from build123d import *

# Parameters (mm, degrees)
F0_R     = 12.7
F1_DEPTH = 6.35
F0_W     = 1.27
F0_H     = 1.27
F2_DEPTH = 2.794


with BuildPart() as f1:
    # F0 (on Front) → F1 (new body, symmetric)
    with BuildSketch(Plane.XZ):
        Circle(F0_R)
        with BuildLine():
            ThreePointArc((8.1567226875, 1.27), (8.2303939998, 0.636898428), (8.255, 0))
            ThreePointArc((8.255, 0), (8.2303939998, -0.636898428), (8.1567226875, -1.27))
            ThreePointArc((8.1567226875, -1.27), (5.8371664787, -5.8371664787), (1.27, -8.1567226875))
            ThreePointArc((1.27, -8.1567226875), (0.636898428, -8.2303939998), (0, -8.255))
            ThreePointArc((0, -8.255), (-0.636898428, -8.2303939998), (-1.27, -8.1567226875))
            ThreePointArc((-1.27, -8.1567226875), (-5.8371664787, -5.8371664787), (-8.1567226875, -1.27))
            ThreePointArc((-8.1567226875, -1.27), (-8.2303939998, -0.636898428), (-8.255, 0))
            ThreePointArc((-8.255, 0), (-8.2303939998, 0.636898428), (-8.1567226875, 1.27))
            ThreePointArc((-8.1567226875, 1.27), (-5.8371664787, 5.8371664787), (-1.27, 8.1567226875))
            ThreePointArc((-1.27, 8.1567226875), (-0.636898428, 8.2303939998), (0, 8.255))
            ThreePointArc((0, 8.255), (0.636898428, 8.2303939998), (1.27, 8.1567226875))
            ThreePointArc((1.27, 8.1567226875), (5.8371664787, 5.8371664787), (8.1567226875, 1.27))
        make_face(mode=Mode.SUBTRACT)
    extrude(amount=F1_DEPTH, both=True)

    # F0 (on Front) → F2 (join, symmetric)
    with BuildSketch(Plane.XZ):
        with BuildLine():
            Line((1.27, 1.27), (1.27, 8.1567226875))
            ThreePointArc((1.27, 8.1567226875), (0.636898428, 8.2303939998), (0, 8.255))
            Line((0, 8.255), (0, 1.27))
            Line((0, 1.27), (1.27, 1.27))
        make_face()
        with BuildLine():
            Line((0, 1.27), (0, 8.255))
            ThreePointArc((0, 8.255), (-0.636898428, 8.2303939998), (-1.27, 8.1567226875))
            Line((-1.27, 8.1567226875), (-1.27, 1.27))
            Line((-1.27, 1.27), (0, 1.27))
        make_face()
        with Locations((-0.635, 0.635)):
            Rectangle(F0_W, F0_H)
        with Locations((0.635, 0.635)):
            Rectangle(F0_W, F0_H)
        with Locations((0.635, -0.635)):
            Rectangle(F0_W, F0_H)
        with Locations((-0.635, -0.635)):
            Rectangle(F0_W, F0_H)
        with BuildLine():
            ThreePointArc((-1.27, -8.1567226875), (-0.636898428, -8.2303939998), (0, -8.255))
            Line((0, -8.255), (0, -1.27))
            Line((0, -1.27), (-1.27, -1.27))
            Line((-1.27, -1.27), (-1.27, -8.1567226875))
        make_face()
        with BuildLine():
            ThreePointArc((0, -8.255), (0.636898428, -8.2303939998), (1.27, -8.1567226875))
            Line((1.27, -8.1567226875), (1.27, -1.27))
            Line((1.27, -1.27), (0, -1.27))
            Line((0, -1.27), (0, -8.255))
        make_face()
        with BuildLine():
            Line((-8.255, 0), (-1.27, 0))
            Line((-1.27, 0), (-1.27, 1.27))
            Line((-1.27, 1.27), (-8.1567226875, 1.27))
            ThreePointArc((-8.1567226875, 1.27), (-8.2303939998, 0.636898428), (-8.255, 0))
        make_face()
        with BuildLine():
            Line((-1.27, -1.27), (-1.27, 0))
            Line((-1.27, 0), (-8.255, 0))
            ThreePointArc((-8.255, 0), (-8.2303939998, -0.636898428), (-8.1567226875, -1.27))
            Line((-8.1567226875, -1.27), (-1.27, -1.27))
        make_face()
        with BuildLine():
            ThreePointArc((8.1567226875, -1.27), (8.2303939998, -0.636898428), (8.255, 0))
            Line((8.255, 0), (1.27, 0))
            Line((1.27, 0), (1.27, -1.27))
            Line((1.27, -1.27), (8.1567226875, -1.27))
        make_face()
        with BuildLine():
            Line((1.27, 0), (8.255, 0))
            ThreePointArc((8.255, 0), (8.2303939998, 0.636898428), (8.1567226875, 1.27))
            Line((8.1567226875, 1.27), (1.27, 1.27))
            Line((1.27, 1.27), (1.27, 0))
        make_face()
    extrude(amount=F2_DEPTH, both=True)


solid = f1.part
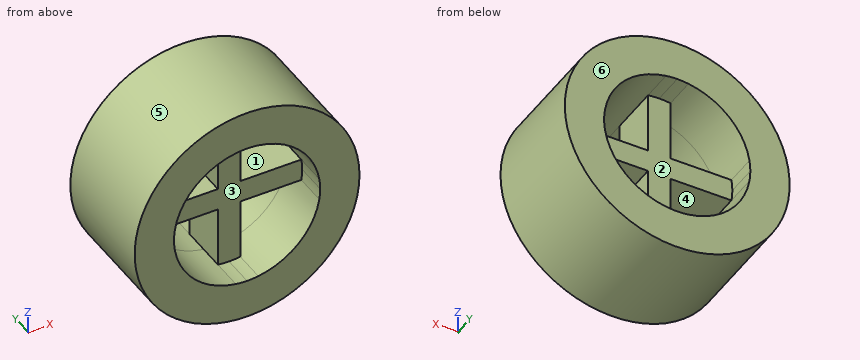
For this review, take the finished solid that the model builds, in its own axes (mm). Face numbers are marked on the shaded views. A direction names the side the tool comes from. Round coordinates to 2 decimals unless told otherwise and drop trailing zeros. Loops run counter-clockwise (first coordinate to the right, second up) from the corner with the lowest first, then second, coordinate; pieces in that order, holes last. Notation, with made-up numbers: (31.5, -32) - (83.5, -32) arc R36 cw to (83.5, 7) - close; hole circle Ø8 at (74.5, 8). An arc over 180 degrees is marked (long way). Use one line per item in the form item = value.
Item 1: Mouldability with a two-part tool opening along Z and no side actions: class the marked faces 4, 5 and 6 as +Z half, -Z half, draft (parallel to the pull), parting line (faces both ways), or undercut.
Answers:
face_4 = undercut
face_5 = parting line
face_6 = draft
Item 2: Consider section B-B on x = 2.5. Write out the cut boundary in (y, z), then the cut area to 3 significant figures.
Answers:
outline = (-6.35, -12.45) - (6.35, -12.45) - (6.35, -7.87) - (-6.35, -7.87) - close; (-6.35, 7.87) - (6.35, 7.87) - (6.35, 12.45) - (-6.35, 12.45) - close; (-2.79, -1.27) - (2.79, -1.27) - (2.79, 1.27) - (-2.79, 1.27) - close
area = 131 mm^2
Item 3: Clearance check with flat-ended pins moving along their axes: P1, Ø4, axis at x = -1, z = 1, coming from the +Y side; P2, Ø4.5, axis at y = 1, z = 3.5, coming from the -X side; P3, Ø1, axis at x = -2.5, y = 3.5, coming from the -Z side. State where each tip first meets the part, or that it passes through.
Answers:
P1 = 2.79
P2 = -12.64
P3 = -12.54
Item 4: For line 1 (X direction, y = -0.25, z = 3.25); line 2 (Y direction, x = -4.5, z = -0.5); line 3 (X direction, y = 4.25, z = -1), list the stretches that pass through material, from the lowest coordinate up.
Answers:
line_1 = -12.28 to -7.59, -1.27 to 1.27, 7.59 to 12.28
line_2 = -2.79 to 2.79
line_3 = -12.66 to -8.19, 8.19 to 12.66
Item 5: Consider section C-C on y = 1. Write out the cut boundary in (x, z) (3 decimals).
Answers:
outline = circle Ø25.4 at (0, 0); hole (-8.157, -1.27) arc R8.255 ccw to (-1.27, -8.157) - (-1.27, -1.27) - close; hole (-8.157, 1.27) - (-1.27, 1.27) - (-1.27, 8.157) arc R8.255 ccw to start; hole (1.27, -8.157) arc R8.255 ccw to (8.157, -1.27) - (1.27, -1.27) - close; hole (1.27, 1.27) - (8.157, 1.27) arc R8.255 ccw to (1.27, 8.157) - close
Item 6: Consider section D-D on z = -7.75. Write out the cut boundary in (x, y).
Answers:
outline = (-10.06, -6.35) - (-2.84, -6.35) - (-2.84, 6.35) - (-10.06, 6.35) - close; (-1.27, -2.79) - (1.27, -2.79) - (1.27, 2.79) - (-1.27, 2.79) - close; (2.84, -6.35) - (10.06, -6.35) - (10.06, 6.35) - (2.84, 6.35) - close
Item 7: Consider section A-A on y = 4.75. Write out the cut boundary in (x, z) (3 decimals).
Answers:
outline = circle Ø25.4 at (0, 0); hole circle Ø16.51 at (0, 0)
Item 8: Tool access review of the marked faces 1, 2 and 3: name each direction out of +Z, -Z, +X, -X, +Y, -Y from which nothing blocks a thin tool from reaching the whole face with its end or side.
Answers:
face_1 = +Y, -Y
face_2 = +Y
face_3 = -Y
